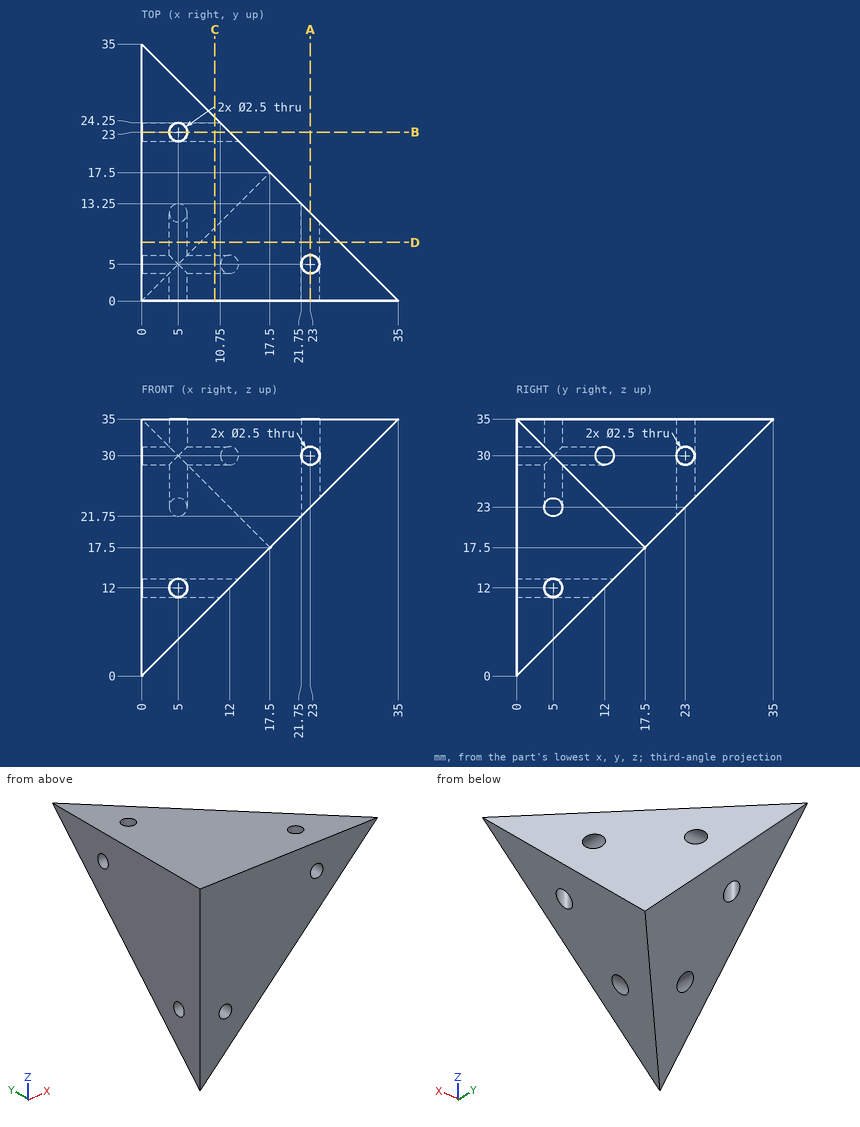
Study the drawing (mm; zero at the part's minimum x, y, z) and answer. Coordinates: 2 decimals unless noted, no trailing zeros. Loops run counter-clockwise (first coordinate to the right, second up) from the corner with the lowest first, then second, coordinate; pieces in that order, holes last. Notation, with made-up numbers: M -30.75,-35 L -12.75,-35 A19 ccw -12.75,-23 Z; hole C 11,-29 d5. An arc over 180 degrees is marked long. Answer as a JSON object with one key per item and string values. Group by question number.
Item 1: Section A-A (x = 23) is taken. Write down the section's boundary in (y, z).
Item 2: Each of these flat-tipped pins is pushed along its axis until it touches: P1, Ø10, axis at x = 14.5, y = 26, coming from the -Z side; P2, Ø4, axis at y = 23, z = 30, coming from the +X side; P3, Ø4, axis at y = 7.5, z = 24, coming from the +X side. Where does it stop, or does it pass through?
Item 3: Consider L1, parallel to Y at x = 5, z = 33; L2, parallel to X at y = 6, z = 30.5; L3, parallel to Y at x = 5.5, z = 25.5. Determine where each line is inside the solid, lowest interval first.
Item 4: Section C-C (x = 10) is taken. Write down the section's boundary in (y, z).
Item 5: Section D-D (y = 8) is taken. Write down the section's boundary in (x, z).
Solved:
{
 "1": {"outline": "M 0,23 L 3.75,23 L 3.75,28.75 L 0,28.75 Z; M 0,31.25 L 3.75,31.25 L 3.75,35 L 0,35 Z; M 6.25,23 L 12,23 L 12,28.75 L 6.25,28.75 Z; M 6.25,31.25 L 12,31.25 L 12,35 L 6.25,35 Z"},
 "2": {"P1": "stops at z = 21.03", "P2": "stops at x = 14", "P3": "stops at x = 26"},
 "3": {"L1": "y = 0 to 21.75, 24.25 to 30", "L2": "x = 0 to 21.85, 24.15 to 29", "L3": "y = 0 to 21.85, 24.15 to 25.5"},
 "4": {"outline": "M 0,10 L 10,10 L 25,25 L 25,35 L 0,35 Z; hole C 5,12 d2.5; hole C 23,30 d2.5"},
 "5": {"outline": "M 0,8 L 8,8 L 27,27 L 27,35 L 0,35 Z; hole C 5,12 d2.5; hole C 23,30 d2.5"}
}
